Source: CAD feature listing. Evaluate the final solid. Frame: model axes, mm. Give positions to 0.01 mm unless a question says otherwise; leave off trailing zeros. Write each loop counter-clockwise with the first axis right and the second up, starting at its lowest first coordinate (ties: lowest second). Pieces come first, ordered by that corner, then holes. Notation, with made-up numbers: (19, -18.5) - (60, -18.5) arc R13 cw to (60, -5.5) - close; hole circle Ø8 at (-13.75, -15.75). An arc over 180 degrees is marked (long way). Answer as a JSON object with one key per item and string values. Group by question number.
from build123d import *

# Parameters (mm, degrees)
F0_W     = 138.9888
F0_H     = 419.989
F1_DEPTH = 5.08
F3_D     = 7.874


with BuildPart() as f1:
    # F0 (on Top) → F1 (new body)
    with BuildSketch(Plane.XY):
        with Locations((69.4944, 309.9943)):
            Rectangle(F0_W, F0_H)
        Polygon((0, 619.9886), (0, 519.9888), (138.9888, 519.9888), (759.0028, 519.9888), (897.9916, 519.9888), (897.9916, 619.9886), align=None)
        with Locations((828.4972, 309.9943)):
            Rectangle(F0_W, F0_H)
        Polygon((0, 99.9998), (0, 0), (897.9916, 0), (897.9916, 99.9998), (759.0028, 99.9998), (138.9888, 99.9998), align=None)
    extrude(amount=F1_DEPTH)

    # F3 (through all)
    with Locations(Plane.XY.offset(5.08)):
        with Locations((108.9914, 539.9786), (124.0028, 554.99), (174.0154, 554.99), (124.0028, 579.9836), (224.028, 579.9836), (224.028, 554.99), (274.0406, 554.99), (324.0532, 579.9836), (324.0532, 554.99), (374.0658, 554.99), (424.0784, 579.9836), (424.0784, 554.99), (474.091, 579.9836), (474.091, 554.99), (524.1036, 554.99), (574.1162, 579.9836), (574.1162, 554.99), (624.1288, 554.99), (674.1414, 579.9836), (674.1414, 554.99), (789.0002, 539.9786), (774.1666, 579.9836), (774.1666, 554.99), (724.154, 554.99), (789.0002, 480.1108), (813.9938, 465.074), (789.0002, 130.0226), (813.9938, 145.034), (789.0002, 180.0352), (789.0002, 230.0478), (813.9938, 225.044), (789.0002, 280.0604), (813.9938, 305.054), (789.0002, 330.073), (789.0002, 380.0856), (813.9938, 385.064), (789.0002, 430.0982), (789.0002, 80.01), (774.1666, 64.9986), (774.1666, 40.005), (724.154, 64.9986), (674.1414, 64.9986), (674.1414, 40.005), (83.9978, 465.074), (108.9914, 480.1108), (108.9914, 430.0982), (83.9978, 385.064), (108.9914, 380.0856), (108.9914, 330.073), (83.9978, 305.054), (108.9914, 280.0604), (83.9978, 225.044), (108.9914, 230.0478), (108.9914, 180.0352), (83.9978, 145.034), (108.9914, 130.0226), (108.9914, 80.01), (124.0028, 64.9986), (124.0028, 40.005), (174.0154, 64.9986), (224.028, 40.005), (224.028, 64.9986), (274.0406, 64.9986), (324.0532, 40.005), (324.0532, 64.9986), (374.0658, 64.9986), (424.0784, 64.9986), (424.0784, 40.005), (474.091, 64.9986), (474.091, 40.005), (524.1036, 64.9986), (574.1162, 64.9986), (624.1288, 64.9986), (574.1162, 40.005)):
            Hole(F3_D / 2)


solid = f1.part
Q1. Section B-B on z = 1.35. State how many separate pieces and enclosed holes the cut face has, then the cut area to 3 significant figures.
Q2. Section A-A on y = 404. Return the cut outline in (x, z), then the cut area to 3 significant figures.
Q3. Ray query, probe 1 along X at (y, z) = (380.5, 4.05); probe 2 along X at (y, z) = (81, 3.4); probe 3 along Y at (x, z) = (245, 4.8). Return the intervals inside material, ascending. Write a range as [from, to].
Taken from the geometry:
{
 "1": {"separate pieces": "1", "enclosed holes": "75", "area": "293,000 mm²"},
 "2": {"outline": "(0, 0) - (138.99, 0) - (138.99, 5.08) - (0, 5.08) - close; (759, 0) - (897.99, 0) - (897.99, 5.08) - (759, 5.08) - close", "area": "1,410 mm²"},
 "3": {"probe 1": "x = [0, 105.08], [112.91, 138.99], [759, 785.09], [792.92, 897.99]", "probe 2": "x = [0, 105.18], [112.8, 785.19], [792.81, 897.99]", "probe 3": "y = [0, 100], [519.99, 619.99]"}
}
